Design review of the part built by this model. Coordinates are the model's own, in mm. A direction names the side the tool comes from. Coordinates: 2 decimals unless noted, no trailing zeros. Loops run counter-clockwise (first coordinate to the right, second up) from the corner with the lowest first, then second, coordinate; pieces in that order, holes last. Notation, with made-up numbers: M -33.5,74.5 L -15.5,74.5 A30 cw -15.5,97.5 Z; hole C -26,-25 d5. An arc over 180 degrees is marked long. Answer as a JSON object with one key per item and string values. Group by question number.
1. To check wall thickness, follow probe 1 along Y at (x, z) = (-11.25, 11.25); probe 2 along X at (y, z) = (0, 7); probe 3 along X at (y, z) = (45, 11.5) (3 decimals). State the ranges of each line that lie inside material, in increasing order.
2. Consider section C-C (y = 85). State the section outline as (x, z) points (3 decimals), then the cut area to 3 significant figures.
3. Consider section D-D (x = 11.25). State the section outline as (y, z) points, then the cut area to 3 significant figures.
4. Consider section B-B (x = 0). State the section outline as (y, z) points.
5. Consider section A-A (z = 10.25). State the section outline as (x, y) points (3 decimals), then the cut area to 3 significant figures.
6. Draft analysis for pull direction X (two halves, no side actions). For faces 4 (the flat face through (0, 17, 10)), 5 (the cylindrical face through (0.969, -29.984, 9.392)), 6 (the flat face through (22.225, 58, 9)), 7 (the flat face through (0, 33, 0)), state which applies: +X half, -X half, draft (parallel to the pull), parting line (faces both ways), or undercut.
7. Machinability: for faces 1 (the flat face through (0, 95.151, 9)), 2 (the flat face through (-22.225, 57, 9)), 3 (the flat face through (-2.5, 16, 10)), which of the approach directions +Z, -Z, +X, -X, +Y, -Y give a long, thin tool a straight path to every point of the face, cutting with its end or side? Answer none if there is none.
8. Insertion check: pin 1 (4 mm diameter, centred on y = 49.5, z = 14.5, fed in from +X) (3 decimals); pin 2 (6 mm diameter, centred on y = 11.5, z = 6.5, fed in from +X); pin 3 (4 mm diameter, centred on x = 11.25, y = 50, fed in from -Z); pin 4 (6 mm diameter, centred on x = -11.25, y = 50, fed in from +Z). Each pin has a flat end and moves straight along its axis. Give the tip position at first contact, or say it passes through.
from build123d import *

# Parameters (mm, degrees)
SKETCH1_R           = 15
BOSS_EXTRUDE1_DEPTH = 19.05
SKETCH2_W           = 5
SKETCH2_H           = 17
CUT_EXTRUDE1_DEPTH  = 102.570428297
SKETCH3_R           = 2.5
CUT_EXTRUDE2_DEPTH  = 102.570428297


with BuildPart() as part:
    # Sketch1 → Boss-Extrude1 (new body)
    with BuildSketch(Plane.XY):
        with BuildLine():
            Line((-22.225, 20.150666862), (-22.225, 95.150666862))
            Line((-22.225, 95.150666862), (22.225, 95.150666862))
            Line((22.225, 95.150666862), (22.225, 20.150666862))
            ThreePointArc((22.225, 20.150666862), (0, -30), (-22.225, 20.150666862))
        make_face()
        with Locations(Location((0, 0, 0), (0, 0, 180))):
            Circle(SKETCH1_R, mode=Mode.SUBTRACT)
    extrude(amount=BOSS_EXTRUDE1_DEPTH)

    # Sketch2 → Cut-Extrude1 (cut, through all)
    with BuildSketch(Plane.XY.offset(19.05)):
        with Locations((0, 8.5)):
            Rectangle(SKETCH2_W, SKETCH2_H)
    extrude(amount=-CUT_EXTRUDE1_DEPTH, mode=Mode.SUBTRACT)

    # Sketch3 → Cut-Extrude2 (cut, through all)
    with BuildSketch(Plane.XY.offset(19.05)):
        with Locations((-11.25, 85)):
            Circle(SKETCH3_R)
        with Locations((11.25, 85)):
            Circle(SKETCH3_R)
        with Locations((11.25, 50)):
            Circle(SKETCH3_R)
        with Locations((-11.25, 50)):
            Circle(SKETCH3_R)
    extrude(amount=-CUT_EXTRUDE2_DEPTH, mode=Mode.SUBTRACT)


solid = part.part
Findings below:
{
 "1": {"probe 1": "y = -27.81 to -9.92, 9.92 to 47.5, 52.5 to 82.5, 87.5 to 95.15", "probe 2": "x = -30 to -15, 15 to 30", "probe 3": "x = -22.225 to 22.225"},
 "2": {"outline": "M -22.225,0 L -13.75,0 L -13.75,19.05 L -22.225,19.05 Z; M -8.75,0 L 8.75,0 L 8.75,19.05 L -8.75,19.05 Z; M 13.75,0 L 22.225,0 L 22.225,19.05 L 13.75,19.05 Z", "area": "656 mm^2"},
 "3": {"outline": "M -27.81,0 L -9.92,0 L -9.92,19.05 L -27.81,19.05 Z; M 9.92,0 L 47.5,0 L 47.5,19.05 L 9.92,19.05 Z; M 52.5,0 L 82.5,0 L 82.5,19.05 L 52.5,19.05 Z; M 87.5,0 L 95.15,0 L 95.15,19.05 L 87.5,19.05 Z", "area": "1,770 mm^2"},
 "4": {"outline": "M -30,0 L -15,0 L -15,19.05 L -30,19.05 Z; M 17,0 L 95.15,0 L 95.15,19.05 L 17,19.05 Z"},
 "5": {"outline": "M -22.225,20.151 A30 ccw long 22.225,20.151 L 22.225,95.151 L -22.225,95.151 Z; hole C -11.25,50 d5; hole C -11.25,85 d5; hole M -2.5,14.79 A15 ccw long 2.5,14.79 L 2.5,17 L -2.5,17 Z; hole C 11.25,50 d5; hole C 11.25,85 d5", "area": "5,060 mm^2"},
 "6": {"face 4": "undercut", "face 5": "parting line", "face 6": "+X half", "face 7": "draft"},
 "7": {"face 1": "+Z, -Z, +X, -X, +Y", "face 2": "+Z, -Z, -X, +Y", "face 3": "+Z, -Z"},
 "8": {"pin 1": "stops at x = 22.225", "pin 2": "stops at x = 28.77", "pin 3": "passes through", "pin 4": "stops at z = 19.05"}
}
